from build123d import *

# Parameters (mm, degrees)
CUT_EXTRUDE2_START  = 500
SKETCH3_R           = 96.25
CUT_EXTRUDE2_DEPTH  = 427.5
CIRPATTERN4_COUNT   = 4
SHELL2_T            = -7.5
SKETCH3_3_R         = 12.5
SKETCH3_3_R_2       = 3.125
CUT_EXTRUDE3_DEPTH  = 141.629166605
CIRPATTERN5_COUNT   = 4
BOSS_EXTRUDE1_START = -50
SKETCH5_R           = 40
SKETCH5_R_2         = 3.125
BOSS_EXTRUDE1_DEPTH = 10


with BuildPart() as part:
    # Main Revolve Sketch → Main Revolve (revolve)
    with BuildSketch(Plane.XY, mode=Mode.PRIVATE) as main_revolve_sk:
        with BuildLine():
            Line((0, 0), (0, 96.25))
            ThreePointArc((0, 96.25), (-58.336309448, 72.086309448), (-82.5, 13.75))
            Line((-82.5, 13.75), (-82.5, 0))
            Line((-82.5, 0), (-82.5, -13.75))
            ThreePointArc((-82.5, -13.75), (-80.374954989, -32.354209486), (-74.109294289, -50))
            Line((-74.109294289, -50), (0, -50))
            Line((0, -50), (0, 0))
        make_face()
    revolve(main_revolve_sk.sketch.rotate(Axis((0, 0, 0), (0, 1, 0)), 270), axis=Axis((0, 0, 0), (0, 1, 0)))

    # Sketch3 → Cut-Extrude2 (cut)
    with BuildSketch(Plane.XY.offset(CUT_EXTRUDE2_START)):
        Circle(SKETCH3_R)
    cut_extrude2 = extrude(amount=-CUT_EXTRUDE2_DEPTH, mode=Mode.SUBTRACT)

    # CirPattern4: Cut-Extrude2 ×4 about axis
    cirpattern4_axis = Axis((0, 0, 0), (0, 1, 0))
    for i in range(1, CIRPATTERN4_COUNT):
        add(cut_extrude2.rotate(cirpattern4_axis, i * 360 / CIRPATTERN4_COUNT), mode=Mode.SUBTRACT)

    # Shell2
    shell2_openings = [part.faces().sort_by_distance(p)[0] for p in [
        (0, -50, 0),
    ]]
    offset(amount=SHELL2_T, openings=shell2_openings)

    # Sketch3<3> → Cut-Extrude3 (cut, through all)
    with BuildSketch(Plane.XY):
        Circle(SKETCH3_3_R)
        with Locations((0, 31.25)):
            Circle(SKETCH3_3_R_2)
        with Locations((27.063293868, 15.625)):
            Circle(SKETCH3_3_R_2)
        with Locations((27.063293868, -15.625)):
            Circle(SKETCH3_3_R_2)
        with Locations((0, -31.25)):
            Circle(SKETCH3_3_R_2)
        with Locations((-27.063293868, -15.625)):
            Circle(SKETCH3_3_R_2)
        with Locations((-27.063293868, 15.625)):
            Circle(SKETCH3_3_R_2)
    cut_extrude3 = extrude(amount=-CUT_EXTRUDE3_DEPTH, mode=Mode.SUBTRACT)

    # CirPattern5: Cut-Extrude3 ×4 about axis
    cirpattern5_axis = Axis((0, 0, 0), (0, -1, 0))
    for i in range(1, CIRPATTERN5_COUNT):
        add(cut_extrude3.rotate(cirpattern5_axis, i * 360 / CIRPATTERN5_COUNT), mode=Mode.SUBTRACT)

    # Sketch5 → Boss-Extrude1 (add)
    with BuildSketch(Plane(origin=(0, 0, 0), x_dir=(1, 0, 0), z_dir=(0, 1, 0)).offset(BOSS_EXTRUDE1_START)):
        with BuildLine():
            Line((-72.5, 15.360257159), (-72.5, -15.360257159))
            ThreePointArc((-72.5, -15.360257159), (-52.403184541, -52.403184541), (-15.360257159, -72.5))
            Line((-15.360257159, -72.5), (15.360257159, -72.5))
            ThreePointArc((15.360257159, -72.5), (52.403184541, -52.403184541), (72.5, -15.360257159))
            Line((72.5, -15.360257159), (72.5, 15.360257159))
            ThreePointArc((72.5, 15.360257159), (52.403184541, 52.403184541), (15.360257159, 72.5))
            Line((15.360257159, 72.5), (-15.360257159, 72.5))
            ThreePointArc((-15.360257159, 72.5), (-52.403184541, 52.403184541), (-72.5, 15.360257159))
        make_face()
        with Locations(Location((0, 0, 0), (0, 0, 270))):
            Circle(SKETCH5_R, mode=Mode.SUBTRACT)
        with Locations(Location((0, -47.5, 0), (0, 0, 270))):
            Circle(SKETCH5_R_2, mode=Mode.SUBTRACT)
        with Locations(Location((47.5, 0, 0), (0, 0, 270))):
            Circle(SKETCH5_R_2, mode=Mode.SUBTRACT)
        with Locations(Location((41.13620668, 23.75, 0), (0, 0, 270))):
            Circle(SKETCH5_R_2, mode=Mode.SUBTRACT)
        with Locations(Location((23.75, 41.13620668, 0), (0, 0, 270))):
            Circle(SKETCH5_R_2, mode=Mode.SUBTRACT)
        with Locations(Location((0, 47.5, 0), (0, 0, 270))):
            Circle(SKETCH5_R_2, mode=Mode.SUBTRACT)
        with Locations(Location((-23.75, 41.13620668, 0), (0, 0, 270))):
            Circle(SKETCH5_R_2, mode=Mode.SUBTRACT)
        with Locations(Location((-41.13620668, 23.75, 0), (0, 0, 270))):
            Circle(SKETCH5_R_2, mode=Mode.SUBTRACT)
        with Locations(Location((-47.5, 0, 0), (0, 0, 270))):
            Circle(SKETCH5_R_2, mode=Mode.SUBTRACT)
        with Locations(Location((-41.13620668, -23.75, 0), (0, 0, 270))):
            Circle(SKETCH5_R_2, mode=Mode.SUBTRACT)
        with Locations(Location((41.13620668, -23.75, 0), (0, 0, 270))):
            Circle(SKETCH5_R_2, mode=Mode.SUBTRACT)
        with Locations(Location((-23.75, -41.13620668, 0), (0, 0, 270))):
            Circle(SKETCH5_R_2, mode=Mode.SUBTRACT)
        with Locations(Location((23.75, -41.13620668, 0), (0, 0, 270))):
            Circle(SKETCH5_R_2, mode=Mode.SUBTRACT)
    extrude(amount=BOSS_EXTRUDE1_DEPTH)


solid = part.part
The model under review builds one solid part; all positions refer to its coordinate system, in mm. A direction names the side the tool comes from. Coordinates: 2 decimals unless noted, no trailing zeros. Loops run counter-clockwise (first coordinate to the right, second up) from the corner with the lowest first, then second, coordinate; pieces in that order, holes last.
(1) Insertion check: P1, Ø20, axis at x = 0, y = 0, coming from the -Z side; P2, Ø8, axis at y = 65.5, z = -19.5, coming from the -X side; P3, Ø3, axis at y = 16.5, z = -45, coming from the -X side; P4, Ø4, axis at x = 51.5, z = -19.5, coming from the +Y side. Each pin has a flat end and moves straight along its axis. Give the tip position at first contact, or say it passes through.
Determined:
P1: passes through
P2: stops at x = -64.61
P3: stops at x = -70.05
P4: stops at y = 76.92
(2) Tool access review of faces 1 (the cylindrical face through (26.85, -45.07, -41.54)), 2 (the cylindrical face through (68.7, -28.15, -0.41)), 3 (the flat face through (-1, 16, 65)): name each direction out of +Z, -Z, +X, -X, +Y, -Y from which nothing blocks a thin tool from reaching the whole face with its end or side.
Determined:
face 1: -Y
face 2: +X, -X
face 3: none
(3) Draft analysis for pull direction Y (two halves, no side actions). For faces 4 (the flat face through (1, 14, -72.5)), 5 (the flat face through (65, 16, 1)), state which applies: +Y half, -Y half, draft (parallel to the pull), parting line (faces both ways), or undercut.
Determined:
face 4: draft
face 5: undercut
(4) Wall thickness on L1, parallel to Z at x = 9, y = -15.5; L2, parallel to X at y = -42, z = -1: over which ranges is each line inside the solid? List them lowest first.
Determined:
L1: z = -72.5 to -65, 65 to 72.5
L2: x = -72.5 to -50.46, -44.54 to -39.99, 39.99 to 44.54, 50.46 to 72.5
(5) Consider section A-A, the plane y = 0. Give the number of separate pieces and of enclosed holes in the cut face, plus the area to 3 significant figures.
Determined:
separate pieces: 4
enclosed holes: 0
area: 2,860 mm2
(6) Consider section B-B, the plane z = -57. Give the boundary of the cut face in (x, y).
Determined:
outline: (-59.64, -13.75) arc R59.64 ccw to (-47.36, -50) - (47.36, -50) arc R59.64 ccw to (59.64, -13.75) - (59.64, 13.75) arc R59.64 ccw to (-59.64, 13.75) - close; hole (-48.74, -13.75) arc R48.74 ccw to (-41.07, -40) - (41.07, -40) arc R48.74 ccw to (48.74, -13.75) - (48.74, 13.75) arc R48.74 ccw to (-48.74, 13.75) - close
